Could you check a few things on this model? Use its own coordinates, in mm. A direction names the side the tool comes from. Give positions to 0.01 mm unless a question says otherwise; leave off trailing zeros. Write each loop counter-clockwise with the first axis right and the second up, starting at its lowest first coordinate (ties: lowest second). Pieces come first, ordered by that corner, then holes. Notation, with made-up numbers: (68.5, 28) - (86.5, 28) arc R19 cw to (86.5, 60) - close; hole circle Ø7 at (80, -28). An arc over 180 degrees is marked (long way). Use one line per item in the form item = value.
```python
from build123d import *

# Parameters (mm, degrees)
SKETCH1_R           = 3.175
PUSHER_BASE_DEPTH   = 15
SKETCH3_R           = 1.95
SCREW_HOLE_DEPTH    = 7.5
SKETCH6_W           = 7.5
SKETCH6_H           = 32
PUSHER_HEAD_DEPTH   = 3.75
FILLET1_R           = 6
FILLET5_R           = 6
FILLET6_R           = 6
SKETCH8_W           = 92.5
SKETCH8_H           = 4.5
BOSS_EXTRUDE1_DEPTH = 7.5
FILLET7_R           = 5


with BuildPart() as part:
    # Sketch1 → pusher base (new body)
    with BuildSketch(Plane.XY):
        Polygon((59.166899441, -45.781018283), (51.666899441, -45.781018283), (41.666899441, -45.781018283), (34.166899441, -45.781018283), (34.166899441, -69.281018283), (40.416899441, -69.281018283), (40.416899441, -62.281018283), (52.916899441, -62.281018283), (52.916899441, -69.281018283), (59.166899441, -69.281018283), align=None)
        with Locations((39.416899441, -49.381018283)):
            Circle(SKETCH1_R, mode=Mode.SUBTRACT)
        with Locations((53.916899441, -49.381018283)):
            Circle(SKETCH1_R, mode=Mode.SUBTRACT)
    extrude(amount=PUSHER_BASE_DEPTH)

    # Sketch3 → screw hole (cut)
    with BuildSketch(Plane.XZ.offset(62.281018283)):
        with Locations(Location((46.666899441, 7.5, 0), (0, 0, 270))):
            Circle(SKETCH3_R)
    extrude(amount=-SCREW_HOLE_DEPTH, mode=Mode.SUBTRACT)

    # Sketch6 → pusher head (add, symmetric)
    with BuildSketch(Plane.XY.offset(7.5)):
        with Locations((46.666899441, -29.781018283)):
            Rectangle(SKETCH6_W, SKETCH6_H)
    extrude(amount=PUSHER_HEAD_DEPTH, both=True)

    # Fillet1
    # the kernel refuses this fillet: 6 mm, written as the material it takes off along each edge
    with BuildSketch(Plane(origin=(74.166899441, -45.781018283, 0), x_dir=(0, 0, 1), z_dir=(-1, 0, 0))) as fillet1_piece_1_section:
        with BuildLine():
            CenterArc((FILLET1_R, -FILLET1_R), FILLET1_R, 90, 90)
            Line((0, -FILLET1_R), (0, 0))
            Line((0, 0), (FILLET1_R, 0))
        make_face()
    fillet1_piece_1 = extrude(amount=55, mode=Mode.PRIVATE)
    fillet1_piece_1 = split(fillet1_piece_1, bisect_by=Plane(origin=(62.291899441, -45.824840722, 3.75), z_dir=(0, 0, 1)), keep=Keep.TOP, mode=Mode.PRIVATE)
    fillet1_piece_1 = split(fillet1_piece_1, bisect_by=Plane(origin=(50.416899441, -45.824840722, 4.566140917), z_dir=(1, 0, 0)), keep=Keep.TOP, mode=Mode.PRIVATE)
    add(fillet1_piece_1, mode=Mode.SUBTRACT)
    with BuildSketch(Plane(origin=(74.166899441, -45.781018283, 0), x_dir=(0, 0, 1), z_dir=(-1, 0, 0))) as fillet1_piece_2_section:
        with BuildLine():
            CenterArc((FILLET1_R, -FILLET1_R), FILLET1_R, 90, 90)
            Line((0, -FILLET1_R), (0, 0))
            Line((0, 0), (FILLET1_R, 0))
        make_face()
    fillet1_piece_2 = extrude(amount=55, mode=Mode.PRIVATE)
    fillet1_piece_2 = split(fillet1_piece_2, bisect_by=Plane(origin=(62.291899441, -47.230240291, 3.75), z_dir=(0, 0, -1)), keep=Keep.TOP, mode=Mode.PRIVATE)
    fillet1_piece_2 = split(fillet1_piece_2, bisect_by=Plane(origin=(50.416899441, -47.230240291, 1.136674626), z_dir=(1, 0, 0)), keep=Keep.TOP, mode=Mode.PRIVATE)
    add(fillet1_piece_2, mode=Mode.SUBTRACT)
    with BuildSketch(Plane(origin=(74.166899441, -45.781018283, 0), x_dir=(0, 0, 1), z_dir=(-1, 0, 0))) as fillet1_piece_3_section:
        with BuildLine():
            CenterArc((FILLET1_R, -FILLET1_R), FILLET1_R, 90, 90)
            Line((0, -FILLET1_R), (0, 0))
            Line((0, 0), (FILLET1_R, 0))
        make_face()
    fillet1_piece_3 = extrude(amount=55, mode=Mode.PRIVATE)
    fillet1_piece_3 = split(fillet1_piece_3, bisect_by=Plane(origin=(46.666899441, -47.230240291, 3.75), z_dir=(0, 0, -1)), keep=Keep.TOP, mode=Mode.PRIVATE)
    fillet1_piece_3 = split(fillet1_piece_3, bisect_by=Plane(origin=(50.416899441, -47.230240291, 1.136674626), z_dir=(-1, 0, 0)), keep=Keep.TOP, mode=Mode.PRIVATE)
    fillet1_piece_3 = split(fillet1_piece_3, bisect_by=Plane(origin=(42.916899441, -47.230240291, 1.136674626), z_dir=(1, 0, 0)), keep=Keep.TOP, mode=Mode.PRIVATE)
    add(fillet1_piece_3, mode=Mode.SUBTRACT)
    with BuildSketch(Plane(origin=(74.166899441, -45.781018283, 0), x_dir=(0, 0, 1), z_dir=(-1, 0, 0))) as fillet1_piece_4_section:
        with BuildLine():
            CenterArc((FILLET1_R, -FILLET1_R), FILLET1_R, 90, 90)
            Line((0, -FILLET1_R), (0, 0))
            Line((0, 0), (FILLET1_R, 0))
        make_face()
    fillet1_piece_4 = extrude(amount=55, mode=Mode.PRIVATE)
    fillet1_piece_4 = split(fillet1_piece_4, bisect_by=Plane(origin=(31.041899441, -45.824840722, 3.75), z_dir=(0, 0, 1)), keep=Keep.TOP, mode=Mode.PRIVATE)
    fillet1_piece_4 = split(fillet1_piece_4, bisect_by=Plane(origin=(42.916899441, -45.824840722, 4.566140917), z_dir=(-1, 0, 0)), keep=Keep.TOP, mode=Mode.PRIVATE)
    add(fillet1_piece_4, mode=Mode.SUBTRACT)
    with BuildSketch(Plane(origin=(74.166899441, -45.781018283, 0), x_dir=(0, 0, 1), z_dir=(-1, 0, 0))) as fillet1_piece_5_section:
        with BuildLine():
            CenterArc((FILLET1_R, -FILLET1_R), FILLET1_R, 90, 90)
            Line((0, -FILLET1_R), (0, 0))
            Line((0, 0), (FILLET1_R, 0))
        make_face()
    fillet1_piece_5 = extrude(amount=55, mode=Mode.PRIVATE)
    fillet1_piece_5 = split(fillet1_piece_5, bisect_by=Plane(origin=(31.041899441, -47.230240291, 3.75), z_dir=(0, 0, -1)), keep=Keep.TOP, mode=Mode.PRIVATE)
    fillet1_piece_5 = split(fillet1_piece_5, bisect_by=Plane(origin=(42.916899441, -47.230240291, 1.136674626), z_dir=(-1, 0, 0)), keep=Keep.TOP, mode=Mode.PRIVATE)
    add(fillet1_piece_5, mode=Mode.SUBTRACT)
    with BuildSketch(Plane(origin=(19.166899441, -45.781018283, 15), x_dir=(0, 0, -1), z_dir=(1, 0, 0))) as fillet1_piece_6_section:
        with BuildLine():
            CenterArc((FILLET1_R, -FILLET1_R), FILLET1_R, 90, 90)
            Line((0, -FILLET1_R), (0, 0))
            Line((0, 0), (FILLET1_R, 0))
        make_face()
    fillet1_piece_6 = extrude(amount=55, mode=Mode.PRIVATE)
    fillet1_piece_6 = split(fillet1_piece_6, bisect_by=Plane(origin=(31.041899441, -45.824840722, 11.25), z_dir=(0, 0, -1)), keep=Keep.TOP, mode=Mode.PRIVATE)
    fillet1_piece_6 = split(fillet1_piece_6, bisect_by=Plane(origin=(42.916899441, -45.824840722, 10.433859083), z_dir=(-1, 0, 0)), keep=Keep.TOP, mode=Mode.PRIVATE)
    add(fillet1_piece_6, mode=Mode.SUBTRACT)
    with BuildSketch(Plane(origin=(19.166899441, -45.781018283, 15), x_dir=(0, 0, -1), z_dir=(1, 0, 0))) as fillet1_piece_7_section:
        with BuildLine():
            CenterArc((FILLET1_R, -FILLET1_R), FILLET1_R, 90, 90)
            Line((0, -FILLET1_R), (0, 0))
            Line((0, 0), (FILLET1_R, 0))
        make_face()
    fillet1_piece_7 = extrude(amount=55, mode=Mode.PRIVATE)
    fillet1_piece_7 = split(fillet1_piece_7, bisect_by=Plane(origin=(31.041899441, -47.230240291, 11.25), z_dir=(0, 0, 1)), keep=Keep.TOP, mode=Mode.PRIVATE)
    fillet1_piece_7 = split(fillet1_piece_7, bisect_by=Plane(origin=(42.916899441, -47.230240291, 13.863325374), z_dir=(-1, 0, 0)), keep=Keep.TOP, mode=Mode.PRIVATE)
    add(fillet1_piece_7, mode=Mode.SUBTRACT)
    with BuildSketch(Plane(origin=(19.166899441, -45.781018283, 15), x_dir=(0, 0, -1), z_dir=(1, 0, 0))) as fillet1_piece_8_section:
        with BuildLine():
            CenterArc((FILLET1_R, -FILLET1_R), FILLET1_R, 90, 90)
            Line((0, -FILLET1_R), (0, 0))
            Line((0, 0), (FILLET1_R, 0))
        make_face()
    fillet1_piece_8 = extrude(amount=55, mode=Mode.PRIVATE)
    fillet1_piece_8 = split(fillet1_piece_8, bisect_by=Plane(origin=(50.416899441, -47.230240291, 13.863325374), z_dir=(-1, 0, 0)), keep=Keep.TOP, mode=Mode.PRIVATE)
    fillet1_piece_8 = split(fillet1_piece_8, bisect_by=Plane(origin=(46.666899441, -47.230240291, 11.25), z_dir=(0, 0, 1)), keep=Keep.TOP, mode=Mode.PRIVATE)
    fillet1_piece_8 = split(fillet1_piece_8, bisect_by=Plane(origin=(42.916899441, -47.230240291, 13.863325374), z_dir=(1, 0, 0)), keep=Keep.TOP, mode=Mode.PRIVATE)
    add(fillet1_piece_8, mode=Mode.SUBTRACT)
    with BuildSketch(Plane(origin=(19.166899441, -45.781018283, 15), x_dir=(0, 0, -1), z_dir=(1, 0, 0))) as fillet1_piece_9_section:
        with BuildLine():
            CenterArc((FILLET1_R, -FILLET1_R), FILLET1_R, 90, 90)
            Line((0, -FILLET1_R), (0, 0))
            Line((0, 0), (FILLET1_R, 0))
        make_face()
    fillet1_piece_9 = extrude(amount=55, mode=Mode.PRIVATE)
    fillet1_piece_9 = split(fillet1_piece_9, bisect_by=Plane(origin=(50.416899441, -45.824840722, 10.433859083), z_dir=(1, 0, 0)), keep=Keep.TOP, mode=Mode.PRIVATE)
    fillet1_piece_9 = split(fillet1_piece_9, bisect_by=Plane(origin=(62.291899441, -45.824840722, 11.25), z_dir=(0, 0, -1)), keep=Keep.TOP, mode=Mode.PRIVATE)
    add(fillet1_piece_9, mode=Mode.SUBTRACT)
    with BuildSketch(Plane(origin=(19.166899441, -45.781018283, 15), x_dir=(0, 0, -1), z_dir=(1, 0, 0))) as fillet1_piece_10_section:
        with BuildLine():
            CenterArc((FILLET1_R, -FILLET1_R), FILLET1_R, 90, 90)
            Line((0, -FILLET1_R), (0, 0))
            Line((0, 0), (FILLET1_R, 0))
        make_face()
    fillet1_piece_10 = extrude(amount=55, mode=Mode.PRIVATE)
    fillet1_piece_10 = split(fillet1_piece_10, bisect_by=Plane(origin=(50.416899441, -47.230240291, 13.863325374), z_dir=(1, 0, 0)), keep=Keep.TOP, mode=Mode.PRIVATE)
    fillet1_piece_10 = split(fillet1_piece_10, bisect_by=Plane(origin=(62.291899441, -47.230240291, 11.25), z_dir=(0, 0, 1)), keep=Keep.TOP, mode=Mode.PRIVATE)
    add(fillet1_piece_10, mode=Mode.SUBTRACT)

    # Fillet5
    fillet5_edges = [part.edges().sort_by_distance(p)[0] for p in [
        (46.666899441, -46.218869418, 11.25),
    ]]
    fillet(fillet5_edges, radius=FILLET5_R)

    # Fillet6
    fillet6_edges = [part.edges().sort_by_distance(p)[0] for p in [
        (46.666899441, -46.218869418, 3.75),
    ]]
    fillet(fillet6_edges, radius=FILLET6_R)

    # Sketch8 → Boss-Extrude1 (add)
    with BuildSketch(Plane(origin=(0, 0, 3.75), x_dir=(-1, 0, 0), z_dir=(0, 0, -1))):
        with Locations((3.333100559, -16.031018283)):
            Rectangle(SKETCH8_W, SKETCH8_H)
    extrude(amount=-BOSS_EXTRUDE1_DEPTH)

    # Fillet7
    fillet7_edges = [part.edges().sort_by_distance(p)[0] for p in [
        (50.416899441, -13.781018283, 7.5),
    ]]
    fillet(fillet7_edges, radius=FILLET7_R)


solid = part.part
```
1. If we mould it in two halves opening along Y, with no side actions, what happens to faces 1 (the face through (42.917, -33, 8)), 2 (the face through (47, -54.781, 8)), 3 (the face through (50.417, -33, 8))? For each: pulls with the +Y half, pulls with the -Y half, needs draft (parallel to the pull), parting line crosses it, or undercut.
Response values:
face_1 = undercut
face_2 = pulls with the -Y half
face_3 = needs draft
2. Imagine slicing it at A-A, the plane y = -59.5. List the corners of the cut face in (x, z) for me.
Response values:
outline = (34.17, 0) - (59.17, 0) - (59.17, 15) - (34.17, 15) - close; hole circle Ø3.9 at (46.67, 7.5)
3. If I drill on line 1 (X direction, y = -47, z = 5.5); line 2 (X direction, y = -60, z = 7.5); line 3 (Y direction, x = 40.5, z = 4.5), over which ranges is the centre line in solid material (lowest first)? Write a range as from..to.
Response values:
line_1 = 34.17..37.32, 41.52..51.82, 56.02..59.17
line_2 = 34.17..44.72, 48.62..59.17
line_3 = -62.28..-52.37, -46.4..-45.97, -18.28..-13.78
4. For pin 1 (6 mm diameter, centred on x = -26.5, z = 7, fed in from -Y); pin 2 (3.5 mm diameter, centred on y = -28, z = 7.5, fed in from -X); pin 3 (1.2 mm diameter, centred on x = 45.5, z = 6.5, fed in from -Y), each with a flat end and sliding along its axis, tell me the tip position at first contact or that it passes through.
Response values:
pin_1 = -18.28
pin_2 = 42.92
pin_3 = -62.28
5. Imagine slicing it at D-D, the plane x = 29. List the corners of the cut face in (y, z) for me, and give its area (4 significant figures).
Response values:
outline = (-18.28, 3.75) - (-13.78, 3.75) - (-13.78, 11.25) - (-18.28, 11.25) - close
area = 33.75 mm²
6. Imagine slicing it at B-B, the plane z = 7.5. List the corners of the cut face in (x, y) for me (3 decimals), and give its area (3 significant figures).
Response values:
outline = (-49.583, -18.281) - (42.917, -18.281) - (42.917, -45.781) - (34.167, -45.781) - (34.167, -69.281) - (40.417, -69.281) - (40.417, -62.281) - (44.717, -62.281) - (44.717, -54.781) - (48.617, -54.781) - (48.617, -62.281) - (52.917, -62.281) - (52.917, -69.281) - (59.167, -69.281) - (59.167, -45.781) - (50.417, -45.781) - (50.417, -18.781) arc R5 ccw to (45.417, -13.781) - (-49.583, -13.781) - close; hole circle Ø6.35 at (39.417, -49.381); hole circle Ø6.35 at (53.917, -49.381)
area = 1,060 mm²
7. Which directions (+Z, -Z, +X, -X, +Y, -Y) give clear straight access to the entire face, cutting with the end or side of a thin tool? Please do faces 4 (the face through (44.763, -58.584, 7.923)), 5 (the face through (39, -45.781, 7)), 6 (the face through (55, -45.781, 7)), 7 (the face through (15, -18, 3.75)).
Response values:
face_4 = -Y
face_5 = +Z, -Z, -X
face_6 = +Z, -Z, +X, +Y
face_7 = -Z, +X, -X, +Y
8. Imagine slicing it at C-C, the plane y = -41. List the corners of the cut face in (x, z) for me.
Response values:
outline = (42.92, 3.75) - (50.42, 3.75) - (50.42, 11.25) - (42.92, 11.25) - close
